Build history of the part. All positions in model axes, mm. Face numbers are marked on the shaded views. A direction names the side the tool comes from. Coordinates: 2 decimals unless noted, no trailing zeros. Write each loop counter-clockwise with the first axis right and the second up, starting at its lowest first coordinate (ties: lowest second). Pieces come first, ordered by that corner, then holes. Notation, with made-up numbers: (40, 51) -> (93, 51) arc R13 ccw to (93, 65) -> close; hole circle Ø3 at (32.5, -26). An arc over 180 degrees is marked (long way). Write each question's results on one line, items separated by ' | '. Start each with the question number.
Q1. Saw through at A-A on x = 0. Give the cut face in (y, z).
Q2. Drill centre lines: line 1 (Y direction, x = 0, z = 4.2); line 2 (Z direction, x = -2, y = 2); line 3 (X direction, y = -1.25, z = 1.4). Where is each one in solid material? Low to high.
Q3. Saw through at B-B on z = 1.4. Give the cut face in (x, y), and give its area (3 significant figures).
Q4. Drop flat-ended pins along their axis: pin 1 Ø2.5 at (x, y) = (0, 0) entering from -Z; pin 2 Ø3 at (x, y) = (-0.5, 3.5) entering from +Z. Give the stop position or say it passes through.
Q5. Tool access for the marked faces 1, 2 and 3: list every direction of +Z, -Z, +X, -X, +Y, -Y with a clear straight run to the whole face (end or side of a thin tool).
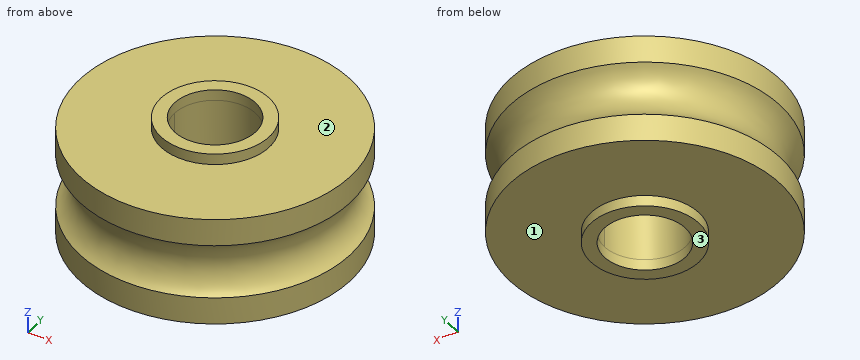
Autodesk Inventor part; units mm, degrees
ref_plane "YZ Plane" through (0, 0, 0) normal (1, 0, 0) x (0, 1, 0)
ref_plane "XZ Plane" through (0, 0, 0) normal (0, 1, 0) x (-1, 0, 0)
ref_plane "XY Plane" through (0, 0, 0) normal (0, 0, 1) x (1, 0, 0)
sketch "Эскиз6" plane through (0, 0, 0) normal (0, 0, 1) x (1, 0, 0)
  circle A0 centre (0, 0) radius 1.5
  circle A1 centre (0, 0) radius 5
  dimension "d16" = 3
  dimension "d30" = 10
extrude "Выдавливание5" add sketch "Эскиз6" along normal blind 4
sketch "Эскиз7" plane through (0, 0, 0) normal (0, 1, 0) x (-1, 0, 0)
  line L0 (0, 0) -> (0, 4)
  line L1 (5, 4) -> (-5, 4)
  line L2 (5, 0) -> (5, 4)
  line L3 (5, 2) -> (4.5, 2)
  line L4 (5, 2) -> (5, 1)
  line L5 (5, 0) -> (5, 4)
  line L6 (5, 1) -> (5, 3)
  line L7 (5, 0) -> (5, 4)
  arc A0 (5, 3) -> (5, 1) centre (5.75, 2) ccw
  point P0 (6.5, 6)
  point P1 (6.5, 0)
  point P2 (5, 3)
  point P3 (5, 1)
  dimension "d31" = 0.5
  dimension "d32" = 1
  dimension "d33" = 2
revolve "Вращение2" cut sketch "Эскиз7" angle 360 about axis through (0, 0, 0) along (0, 0, 1)
fillet "Сопряжение3" [suppressed]
sketch "Эскиз8" plane through (0, 0, 0) normal (0, 0, -1) x (-1, 0, 0)
  circle A0 centre (0, 0) radius 2
  circle A1 centre (0, 0) radius 1.5
  dimension "d25" = 4
extrude "Выдавливание6" add sketch "Эскиз8" along normal blind 0.4 and the other way blind 4.4
properties part number "rolik_2" material "Серебро"
Returned:
1) outline: (-5, 0) -> (-2, 0) -> (-2, -0.4) -> (-1.5, -0.4) -> (-1.5, 4.4) -> (-2, 4.4) -> (-2, 4) -> (-5, 4) -> (-5, 3) arc R1.25 cw to (-5, 1) -> close; (1.5, -0.4) -> (2, -0.4) -> (2, 0) -> (5, 0) -> (5, 1) arc R1.25 cw to (5, 3) -> (5, 4) -> (2, 4) -> (2, 4.4) -> (1.5, 4.4) -> close
2) line 1: y = -2 to -1.5, 1.5 to 2 | line 2: z = 0 to 4 | line 3: x = -4.48 to -0.83, 0.83 to 4.48
3) outline: circle Ø9.31 at (0, 0); hole circle Ø3 at (0, 0) | area: 61.0 mm2
4) pin 1: passes through | pin 2: stops at z = 4
5) face 1: -Z | face 2: +Z | face 3: -Z, +X, -X, +Y, -Y
